```python
from build123d import *

# Parameters (mm, degrees)
SKETCH008_R     = 47.5
PAD004_DEPTH    = 5
SKETCH009_R     = 40
SKETCH009_R_2   = 35
POCKET002_DEPTH = 3
SKETCH015_R     = 1.75
POCKET008_DEPTH = 5
SKETCH022_W     = 13.2
SKETCH022_H     = 2.5
PAD006_DEPTH    = 1


with BuildPart() as part:
    # Sketch008 → Pad004 (new body)
    with BuildSketch(Plane.XY):
        Circle(SKETCH008_R)
    extrude(amount=PAD004_DEPTH)

    # Sketch009 (on Face3 of Pad004) → Pocket002 (cut)
    with BuildSketch(Plane.XY.offset(5)):
        with Locations((-70, 0)):
            Circle(SKETCH009_R)
        with Locations((-70, 0)):
            Circle(SKETCH009_R_2, mode=Mode.SUBTRACT)
    extrude(amount=-POCKET002_DEPTH, mode=Mode.SUBTRACT)

    # Sketch015 (on Face3 of Pocket002) → Pocket008 (cut)
    with BuildSketch(Plane.XY.offset(5)):
        with Locations((-40, 0)):
            Circle(SKETCH015_R)
        with Locations((-12.363995, 38.041183)):
            Circle(SKETCH015_R)
        with Locations((32.356581, 23.51705)):
            Circle(SKETCH015_R)
        with Locations((32.366826, -23.502949)):
            Circle(SKETCH015_R)
        with Locations((-12.347418, -38.046567)):
            Circle(SKETCH015_R)
    extrude(amount=-POCKET008_DEPTH, mode=Mode.SUBTRACT)

    # Sketch022 (on Face3 of Pocket008) → Pad006 (join)
    with BuildSketch(Plane.XY.offset(5)):
        with Locations((0, 34.25)):
            Rectangle(SKETCH022_W, SKETCH022_H)
    extrude(amount=PAD006_DEPTH)


solid = part.part
```
The listing builds one solid part. Answer for the finished solid, in the listing's coordinates (mm). A direction names the side the tool comes from. Coordinates: 2 decimals unless noted, no trailing zeros. Loops run counter-clockwise (first coordinate to the right, second up) from the corner with the lowest first, then second, coordinate; pieces in that order, holes last. Notation, with made-up numbers: (40.25, 72) - (49.25, 72) arc R37 ccw to (49.25, 111) - close; hole circle Ø8 at (61, -3). An arc over 180 degrees is marked (long way). Write item = value, one per line.
1) Section C-C (x = 0) is taken. Determine the outline of the cut face in (y, z), plus the area to 4 significant figures.
Responses:
outline = (-47.5, 0) - (47.5, 0) - (47.5, 5) - (35.5, 5) - (35.5, 6) - (33, 6) - (33, 5) - (-47.5, 5) - close
area = 477.5 mm^2
2) Determine the mould class of faces 1 (the face through (-10.3, -46.37, 2.46)), 2 (the face through (-13.637, -36.864, 2.535)), 3 (the face through (3, 1, 5)) for opening direction X: pulls with the +X half, pulls with the -X half, needs draft (parallel to the pull), parting line crosses it, or undercut.
Responses:
face_1 = parting line crosses it
face_2 = undercut
face_3 = needs draft
3) Find the intervals of material crossed by line 1 along Y through (x, z) = (31.5, 1.8); line 2 along X through (y, z) = (1, 4.3); line 3 along Z through (x, y) = (-12.5, 5), in increasing order.
Responses:
line_1 = -35.55 to -25.02, -21.98 to 21.99, 25.04 to 35.55
line_2 = -47.49 to -41.44, -38.56 to -35.01, -30.01 to 47.49
line_3 = 0 to 5
4) Section B-B (z = 3.4) is taken. Determine the outline of the cut face in (x, y).
Responses:
outline = (-42.37, -21.48) arc R35 ccw to (-42.37, 21.48) arc R47.5 ccw to start; (-39.69, -26.1) arc R47.5 ccw (long way) to (-39.69, 26.1) arc R40 cw to start; hole circle Ø3.5 at (-40, 0); hole circle Ø3.5 at (-12.36, 38.04); hole circle Ø3.5 at (-12.35, -38.05); hole circle Ø3.5 at (32.36, 23.52); hole circle Ø3.5 at (32.37, -23.5)
5) Section A-A (y = 0) is taken. Determine the outline of the cut face in (x, z), plus the area to 4 significant figures.
Responses:
outline = (-47.5, 0) - (-41.75, 0) - (-41.75, 5) - (-47.5, 5) - close; (-38.25, 0) - (47.5, 0) - (47.5, 5) - (-30, 5) - (-30, 2) - (-35, 2) - (-35, 5) - (-38.25, 5) - close
area = 442.5 mm^2
6) Section D-D (y = 13.5) is taken. Determine the outline of the cut face in (x, z), plus the area to 3 significant figures.
Responses:
outline = (-45.54, 0) - (45.54, 0) - (45.54, 5) - (-32.35, 5) - (-32.35, 2) - (-37.71, 2) - (-37.71, 5) - (-45.54, 5) - close
area = 439 mm^2
7) Each of these flat-tipped pins is pushed along its axis until it touches: P1, Ø0.5, axis at x = 1, z = 5.5, coming from the -Y side; P2, Ø13.5, axis at x = -36, y = 1, coming from the +Z side; P3, Ø3, axis at x = -40, y = 0, coming from the +Z side; P4, Ø1.5, axis at y = -34.5, z = 4.5, coming from the +X side. Where does it stop, or does it pass through?
Responses:
P1 = 33
P2 = 5
P3 = through
P4 = 33.42
8) Which of the six approach directions +Z, -Z, +X, -X, +Y, -Y give full straight-line access (tool end or side, diameter ignored) to faces 4 (the face through (30.61, 23.59, 2.54)), 5 (the face through (-30, 0, 4))?
Responses:
face_4 = +Z, -Z
face_5 = +Z
